Geometry: final body of the model. Coordinates: model frame, mm. A direction names the side the tool comes from. Give positions to 0.01 mm unless a question says otherwise; leave off trailing zeros. Write each loop counter-clockwise with the first axis right and the second up, starting at its lowest first coordinate (ties: lowest second). Pieces come first, ordered by that corner, then holes. Notation, with made-up numbers: (18.25, 39.5) -> (48.25, 39.5) arc R25 ccw to (48.25, 72.5) -> close; hole circle Ø7 at (39, 54.5). An arc over 180 degrees is marked (long way). Answer in a Markdown table with one row per item. Add a question column.
Item 1: Section query C-C on z = 2.5. Output: boundary loops of the cut face in (x, y), plus the area to 3 significant figures.
Item 2: First-contact query: P1, Ø6, axis at x = -1.5, y = -13.5, coming from the -Z side; P2, Ø13.5, axis at x = -3, y = 0, coming from the +Z side. Flat tips, straight axial feed; report the tip coordinate or a pass-through.
Item 3: Access query for faces 4 (the cylindrical face through (18.95, -0.26, 1)), 5 (the flat face through (3, 4, 0)). Directions: +Z, -Z, +X, -X, +Y, -Y. A direction counts if a zero-diameter tool reaches every point of the face in a straight line with its end or side. Return the directions, or none.
Item 4: Material intervals for probe 1 along Z at (x, y) = (-1, 1.5); probe 2 along Z at (x, y) = (10, 1.5); probe 3 along X at (y, z) = (-1.5, 15), sorted ascending. Write a range as from..to.
Item 5: Section query D-D on y = -7.5. Output: boundary loops of the cut face in (x, z), plus the area to 3 significant figures.
Item 6: Section query B-B on x = 14. Output: boundary loops of the cut face in (y, z).
Item 7: Draft query along Y for faces 1 (the flat face through (0, 0, 15.9)), 2 (the cylindrical face through (0.26, 19, 14.95)), 3 (the flat face through (-20, 0, 8)). Return one class per face: +Y half, -Y half, draft (parallel to the pull), parting line (faces both ways), or undercut.
Item 8: Section query A-A on y = -2. Output: boundary loops of the cut face in (x, z).
Autodesk Inventor part; units mm, degrees
ref_plane "YZ Plane" through (0, 0, 0) normal (1, 0, 0) x (0, 1, 0)
ref_plane "XZ Plane" through (0, 0, 0) normal (0, 1, 0) x (-1, 0, 0)
ref_plane "XY Plane" through (0, 0, 0) normal (0, 0, 1) x (1, 0, 0)
sketch "Sketch1" plane through (0, 0, 0) normal (0, 0, 1) x (1, 0, 0)
  line L0 (-20, -20) -> (20, -20)
  line L1 (20, -20) -> (20, 20)
  line L2 (20, 20) -> (-20, 20)
  line L3 (-20, 20) -> (-20, -20)
  line L4 (-20, -20) -> (20, 20) construction
  line L5 (20, -20) -> (-20, 20) construction
  point P0 (0, 0)
  dimension "d0" = 40
  dimension "d1" = 40
extrude "Extrusion1" add sketch "Sketch1" along normal blind 16
sketch "Sketch2" plane through (0, 0, 16) normal (0, 0, 1) x (1, 0, 0)
  line L0 (-13.5, -13.5) -> (13.5, -13.5)
  line L1 (13.5, -13.5) -> (13.5, 13.5)
  line L2 (13.5, 13.5) -> (-13.5, 13.5)
  line L3 (-13.5, 13.5) -> (-13.5, -13.5)
  line L4 (-13.5, -13.5) -> (13.5, 13.5) construction
  line L5 (13.5, -13.5) -> (-13.5, 13.5) construction
  point P0 (0, 0)
  dimension "d7" = 27
  dimension "d8" = 27
extrude "Extrusion2" cut sketch "Sketch2" against normal blind 0.1
fillet "Fillet1" radius 2 4 edges at (-13.5, 13.5, 15.95) (13.5, 13.5, 15.95) (13.5, -13.5, 15.95) (-13.5, -13.5, 15.95)
chamfer "Chamfer1" distance 3 angle 45 4 edges at (20, 20, 8) (20, -20, 8) (-20, -20, 8) (-20, 20, 8)
fillet "Fillet2" radius 3.5 8 edges at (20, 0, 16) (0, 20, 16) (0, -20, 16) (-20, 0, 16) (-20, 0, 0) (20, 0, 0) (0, 20, 0) (0, -20, 0)
sketch "Sketch3" plane through (0, 0, 0) normal (0, 0, -1) x (-1, 0, 0)
  circle A0 centre (0, 0) radius 4.25
  dimension "d13" = 8.5
extrude "Extrusion3" add sketch "Sketch3" along normal blind 2
properties part number "LED Light"
Findings below:
| question | item | result |
|---|---|---|
| 1 | outline | (-19.85, -17.15) -> (-17.15, -19.85) -> (17.15, -19.85) -> (19.85, -17.15) -> (19.85, 17.15) -> (17.15, 19.85) -> (-17.15, 19.85) -> (-19.85, 17.15) -> close |
| 1 | area | 1,560 mm^2 |
| 2 | P1 | stops at z = 0 |
| 2 | P2 | stops at z = 15.9 |
| 3 | face 4 | -Z, +X, +Y, -Y |
| 3 | face 5 | -Z |
| 4 | probe 1 | z = -2..15.9 |
| 4 | probe 2 | z = 0..15.9 |
| 4 | probe 3 | x = -18.95..18.95 |
| 5 | outline | (-20, 3.5) arc R3.5 ccw to (-16.5, 0) -> (16.5, 0) arc R3.5 ccw to (20, 3.5) -> (20, 12.5) arc R3.5 ccw to (16.5, 16) -> (13.5, 16) -> (13.5, 15.9) -> (-13.5, 15.9) -> (-13.5, 16) -> (-16.5, 16) arc R3.5 ccw to (-20, 12.5) -> close |
| 5 | area | 627 mm^2 |
| 6 | outline | (-20, 3.5) arc R3.5 ccw to (-16.5, 0) -> (16.5, 0) arc R3.5 ccw to (20, 3.5) -> (20, 12.5) arc R3.5 ccw to (16.5, 16) -> (-16.5, 16) arc R3.5 ccw to (-20, 12.5) -> close |
| 7 | face 1 | undercut |
| 7 | face 2 | +Y half |
| 7 | face 3 | draft |
| 8 | outline | (-20, 3.5) arc R3.5 ccw to (-16.5, 0) -> (-3.75, 0) -> (-3.75, -2) -> (3.75, -2) -> (3.75, 0) -> (16.5, 0) arc R3.5 ccw to (20, 3.5) -> (20, 12.5) arc R3.5 ccw to (16.5, 16) -> (13.5, 16) -> (13.5, 15.9) -> (-13.5, 15.9) -> (-13.5, 16) -> (-16.5, 16) arc R3.5 ccw to (-20, 12.5) -> close |
